```python
from build123d import *

# Parameters (mm, degrees)
F0_W     = 83.26438
F0_H     = 11.269071
F1_DEPTH = 30


with BuildPart() as f1:
    # F0 (on Top) → F1 (new body)
    with BuildSketch(Plane.XY):
        Polygon((51.961524, -30), (51.961524, 30), (0, 60), (-51.961524, 30), (-51.961524, -30), (0, -60), align=None)
        with Locations((-0.318665, -17.973065)):
            Rectangle(F0_W, F0_H, mode=Mode.SUBTRACT)
        with Locations((-0.318665, 3.526934)):
            Rectangle(F0_W, F0_H, mode=Mode.SUBTRACT)
        with Locations((-0.318665, 25.026934)):
            Rectangle(F0_W, F0_H, mode=Mode.SUBTRACT)
    extrude(amount=F1_DEPTH)


solid = f1.part
```
Can you work these out from the model? Positions are in its coordinate system, mm. A direction names the side the tool comes from. Round coordinates to 2 decimals unless told otherwise and drop trailing zeros. Loops run counter-clockwise (first coordinate to the right, second up) from the corner with the lowest first, then second, coordinate; pieces in that order, holes last.
Item 1: Suppose I cut it at A-A, the plane z = 4.5. Write out the boundary of the cut face in (x, y).
Item 2: Will these pins go through, and if not, where does the flat tip stop? pin 1 Ø3 at (y, z) = (39.5, 7.5) entering from +X; pin 2 Ø3 at (x, y) = (13.5, 0.5) entering from +Z; pin 3 Ø12 at (x, z) = (-12, 12.5) entering from -Y; pin 4 Ø6 at (x, z) = (39, 24) entering from +Y.
Item 3: Suppose I cut it at D-D, the plane x = 28. Write out the boundary of the cut face in (y, z), then the cut area to 3 significant figures.
Item 4: Which directions (+Z, -Z, +X, -X, +Y, -Y) give clear straight access to the entire face, cutting with the end or side of a thin tool? Please do faces 1 (the flat face through (-1, -26, 0)), 2 (the flat face through (-41.951, 3, 15)).
Item 5: Suppose I cut it at B-B, the plane y = 1. Write out the boundary of the cut face in (x, z).
Item 6: If we mould it in two halves opening along X, with no side actions, what happens to faces 3 (the flat face through (-25.62, 45.21, 14.79)), 4 (the flat face through (26.344, 44.79, 14.79)), 5 (the flat face through (-41.951, -18, 15)), 6 (the flat face through (41.314, 3, 15))? For each: +X half, -X half, draft (parallel to the pull), parting line (faces both ways), or undercut.
Item 7: Please list where these lines run through material, in increasing order: L1, parallel to Y at x = 10.5, z = 27.5; L2, parallel to X at y = 27, z = 2.25; L3, parallel to Y at x = -27, z = 10.25.
Item 8: Suppose I cut it at C-C, the plane x = -21. Write out the boundary of the cut face in (y, z).
Reported:
1. outline: (-51.96, -30) - (0, -60) - (51.96, -30) - (51.96, 30) - (0, 60) - (-51.96, 30) - close; hole (-41.95, -23.61) - (41.31, -23.61) - (41.31, -12.34) - (-41.95, -12.34) - close; hole (-41.95, -2.11) - (41.31, -2.11) - (41.31, 9.16) - (-41.95, 9.16) - close; hole (-41.95, 19.39) - (41.31, 19.39) - (41.31, 30.66) - (-41.95, 30.66) - close
2. pin 1: stops at x = 38.11
2. pin 2: passes through
2. pin 3: stops at y = -56.54
2. pin 4: stops at y = 39.22
3. outline: (-43.83, 0) - (-23.61, 0) - (-23.61, 30) - (-43.83, 30) - close; (-12.34, 0) - (-2.11, 0) - (-2.11, 30) - (-12.34, 30) - close; (9.16, 0) - (19.39, 0) - (19.39, 30) - (9.16, 30) - close; (30.66, 0) - (43.83, 0) - (43.83, 30) - (30.66, 30) - close
3. area: 1,620 mm2
4. face 1: -Z, +X, -X, +Y, -Y
4. face 2: +Z, -Z
5. outline: (-51.96, 0) - (-41.95, 0) - (-41.95, 30) - (-51.96, 30) - close; (41.31, 0) - (51.96, 0) - (51.96, 30) - (41.31, 30) - close
6. face 3: -X half
6. face 4: +X half
6. face 5: undercut
6. face 6: undercut
7. L1: y = -53.94 to -23.61, -12.34 to -2.11, 9.16 to 19.39, 30.66 to 53.94
7. L2: x = -51.96 to -41.95, 41.31 to 51.96
7. L3: y = -44.41 to -23.61, -12.34 to -2.11, 9.16 to 19.39, 30.66 to 44.41
8. outline: (-47.88, 0) - (-23.61, 0) - (-23.61, 30) - (-47.88, 30) - close; (-12.34, 0) - (-2.11, 0) - (-2.11, 30) - (-12.34, 30) - close; (9.16, 0) - (19.39, 0) - (19.39, 30) - (9.16, 30) - close; (30.66, 0) - (47.88, 0) - (47.88, 30) - (30.66, 30) - close
